Check sheet for the drawn part. Datum: minimum x, y, z corner. Units: mm. A direction names the side the tool comes from. Round coordinates to 2 decimals unless told otherwise and drop trailing zeros. Write each loop counter-clockwise with the first axis right and the second up, starting at its lowest first coordinate (ties: lowest second). Pieces come first, ordered by that corner, then holes. Notation, with made-up numbers: M 47,45.25 L 72,45.25 A13 ccw 72,65.25 Z; hole C 57,53.25 d11. An arc over 180 degrees is marked long. One line per item, written item: value.
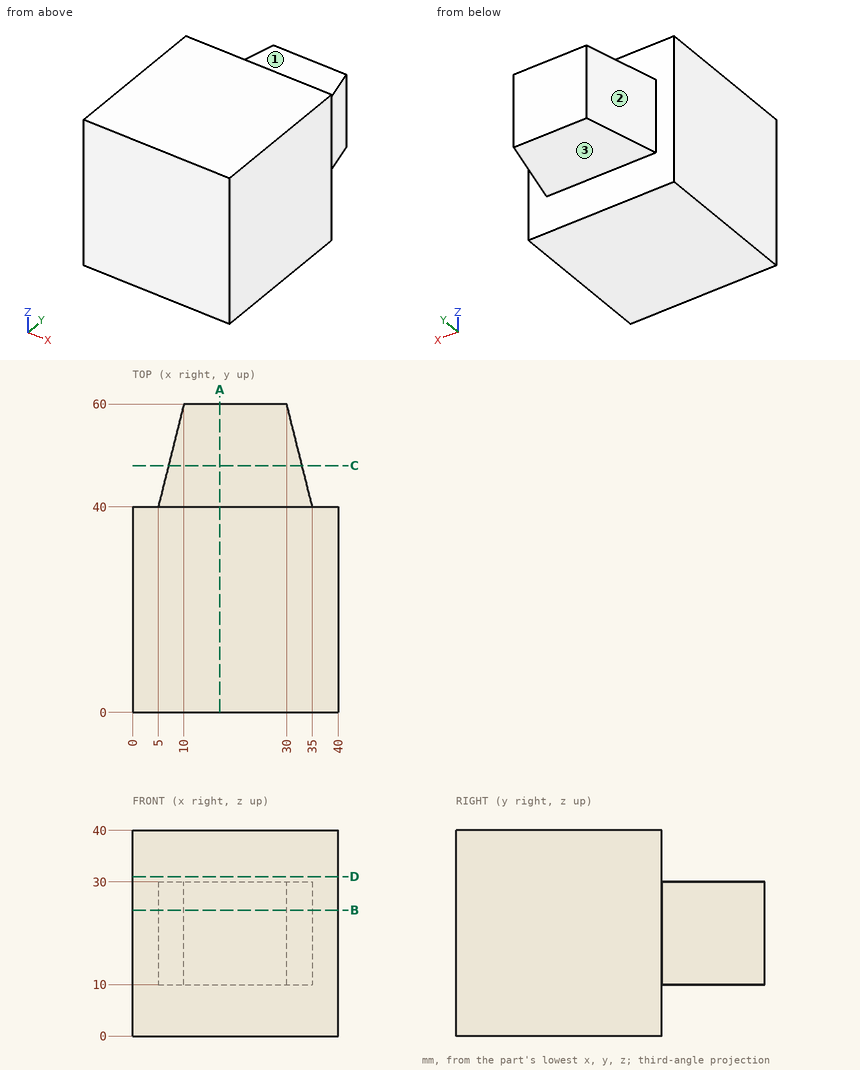
Q1. Sectioned sample at B-B on z = 24.5. Enter the section's corners in (x, y).
Completed:
outline: M 0,0 L 40,0 L 40,40 L 35,40 L 30,60 L 10,60 L 5,40 L 0,40 Z
Q2. Access from +Z, -Z, +X, -X, +Y, -Y to the whole of each face (thin tool, end or side, straight path). Record for the marked faces 1, 2 and 3.
Completed:
face 1: +Z, +X, -X, +Y
face 2: +Z, -Z, -X, +Y
face 3: -Z, +X, -X, +Y
Q3. Sectioned sample at C-C on y = 48. Enter the section's corners in (x, z).
Completed:
outline: M 7,10 L 33,10 L 33,30 L 7,30 Z
Q4. Scan lines: line 1 (Z direction, x = 10, y = 46.5); line 2 (Y direction, x = 38, z = 23.5). Record each from-to range of solid material in increasing order. Write a range as [from, to].
Completed:
line 1: [10, 30]
line 2: [0, 40]
Q5. Sectioned sample at A-A on x = 17. Enter the section's corners in (y, z), and give its area (3 significant figures).
Completed:
outline: M 0,0 L 40,0 L 40,10 L 60,10 L 60,30 L 40,30 L 40,40 L 0,40 Z
area: 2,000 mm^2
Q6. Sectioned sample at D-D on z = 31. Enter the section's corners in (x, y), and give its area (3 significant figures).
Completed:
outline: M 0,0 L 40,0 L 40,40 L 0,40 Z
area: 1,600 mm^2
Q7. Depth check by flat-ended pin: P1, Ø10, axis at x = 16.5, y = 51.5, coming from the +Z side; P2, Ø6, axis at x = 14, y = 47.5, coming from the -Z side; P3, Ø6, axis at x = 14, z = 4.5, coming from the +Y side. Enter the tip coordinate at first touch or a pass-through.
Completed:
P1: z = 30
P2: z = 10
P3: y = 40
